The figure shows three views and two pictorial views of one solid part (mm, origin at its lowest corner). Answer the questions. Coordinates: 2 decimals unless noted, no trailing zeros. Order: outer loops, then holes, each group sorted by start corner. A loop starts at its lowest first (then second) coordinate and runs counter-clockwise, first axis right, second up. Notation, with made-up numbers: M 89,-4.75 L 112,-4.75 A14 cw 112,18.25 Z; hole C 3,-31.75 d2. An arc over 180 degrees is marked long. Answer in a Markdown table with one row per item. Add a question column.
Item 1: The part is cut by section A-A (z = 49). State how many separate pieces and enclosed holes the cut face has, then the cut area to 3 significant figures.
Item 2: Consider line 1 (X direction, y = 103, z = 48); line 2 (Z direction, x = 28, y = 97.5); line 3 (X direction, y = 67.5, z = 77). Determine where each line is inside the solid, lowest interval first. Write a range as from..to.
Item 3: The mould has two halves that part along Z. Classify the marked faces 1 and 2: released by +Z, released by -Z, zero draft, split by the parting line, or undercut.
Item 4: The part is cut by section C-C (z = 67). Write down the section's boundary in (x, y).
Item 5: Flat-ended cylindrical pins translate along their axes: pin 1 Ø1.5 at (y, z) = (92, 12) entering from -X; pin 2 Ø3 at (y, z) = (37.5, 27) entering from -X; pin 3 Ø1.5 at (x, y) = (35.5, 37.5) entering from +Z. Find the tip coordinate at first contact, or state that the pin passes through.
Item 6: The part is cut by section B-B (x = 49). Write down the section's boundary in (y, z).
Item 7: The part is cut by section D-D (y = 52). Write down the section's boundary in (x, z), then the cut area to 3 significant figures.
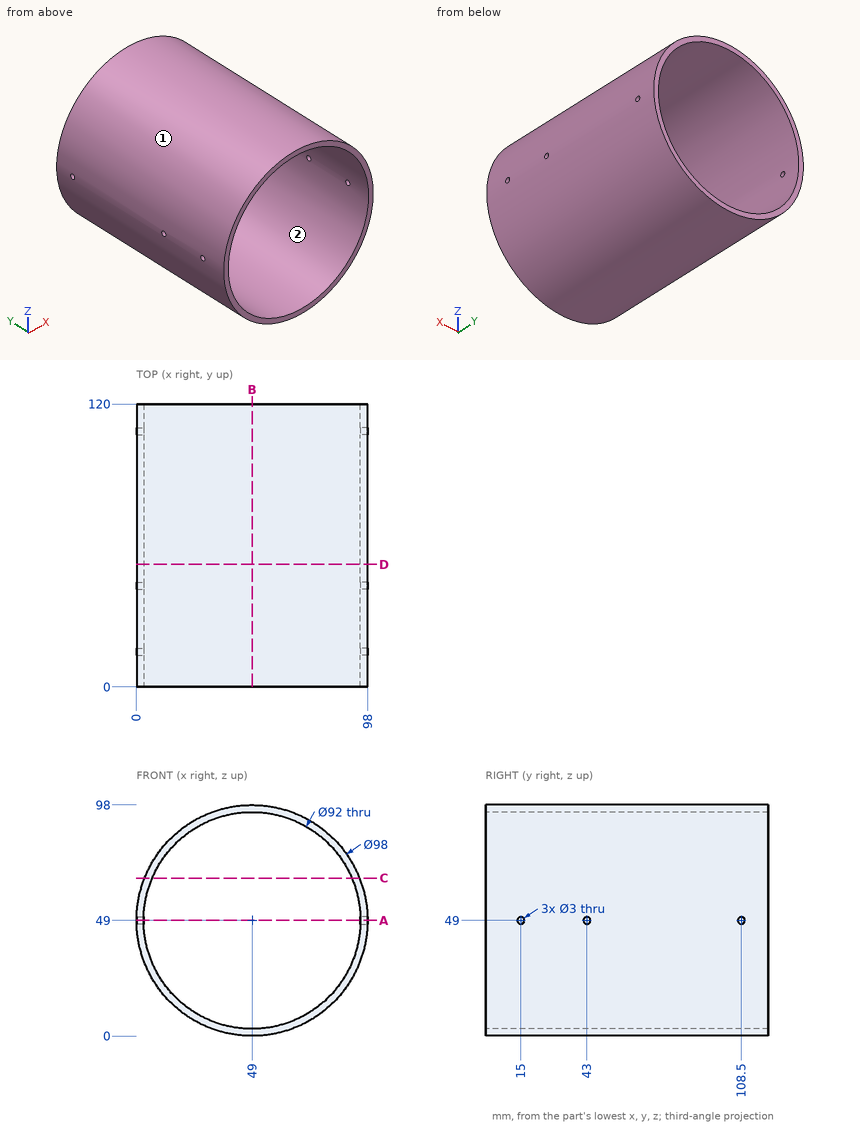
Reply:
| question | item | result |
|---|---|---|
| 1 | separate pieces | 8 |
| 1 | enclosed holes | 0 |
| 1 | area | 666 mm2 |
| 2 | line 1 | x = 0.01..3.01, 94.99..97.99 |
| 2 | line 2 | z = 4.73..8.07, 89.93..93.27 |
| 2 | line 3 | x = 8.79..12.5, 85.5..89.21 |
| 3 | face 1 | split by the parting line |
| 3 | face 2 | undercut |
| 4 | outline | M 3.43,0 L 6.67,0 L 6.67,120 L 3.43,120 Z; M 91.33,0 L 94.57,0 L 94.57,120 L 91.33,120 Z |
| 5 | pin 1 | stops at x = 16.03 |
| 5 | pin 2 | stops at x = 4.49 |
| 5 | pin 3 | stops at z = 96.31 |
| 6 | outline | M 0,0 L 120,0 L 120,3 L 0,3 Z; M 0,95 L 120,95 L 120,98 L 0,98 Z |
| 7 | outline | C 49,49 d98; hole C 49,49 d92 |
| 7 | area | 895 mm2 |
